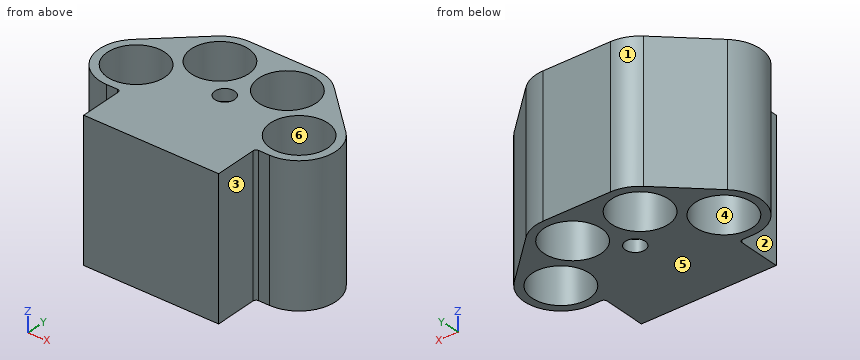
```python
from build123d import *

# Parameters (mm, degrees)
SKETCH1_R           = 7.25
BOSS_EXTRUDE1_DEPTH = 17.5
SKETCH2_R           = 2.5
CUT_EXTRUDE1_DEPTH  = 61.478337768
CUT_EXTRUDE2_START  = -32
SKETCH3_R           = 4
CUT_EXTRUDE2_DEPTH  = 29


with BuildPart() as part:
    # Sketch1 → Boss-Extrude1 (new, symmetric)
    with BuildSketch(Plane.XY):
        with BuildLine():
            ThreePointArc((-20.545709694, 9.528396762), (-29.148813935, 15.380000463), (-26.867170799, 25.531294621))
            Line((-26.867170799, 25.531294621), (-14.821461106, 36.807414431))
            ThreePointArc((-14.821461106, 36.807414431), (-11.898396299, 38.657620814), (-8.5, 39.304516572))
            Line((-8.5, 39.304516572), (0, 39.304516572))
            Line((0, 39.304516572), (0, -2))
            Line((0, -2), (-17, -2))
            Line((-17, -2), (-17, 8.778396762))
            ThreePointArc((-17, 8.778396762), (-17.219669914, 9.308726848), (-17.75, 9.528396762))
            Line((-17.75, 9.528396762), (-20.545709694, 9.528396762))
        make_face()
        with Locations((-8.5, 30.054516572)):
            Circle(SKETCH1_R, mode=Mode.SUBTRACT)
        with Locations((-20.545709694, 18.778396762)):
            Circle(SKETCH1_R, mode=Mode.SUBTRACT)
    boss_extrude1 = extrude(amount=BOSS_EXTRUDE1_DEPTH, both=True)

    # Mirror1: Boss-Extrude1 across plane
    add(boss_extrude1.mirror(Plane(origin=(0, 0, 0), x_dir=(0, 0, 1), z_dir=(1, 0, 0))))

    # Sketch2 → Cut-Extrude1 (cut, through all)
    with BuildSketch(Plane(origin=(0, 0, -17.5), x_dir=(-1, 0, 0), z_dir=(0, 0, -1))):
        with Locations((0, 21)):
            Circle(SKETCH2_R)
    extrude(amount=-CUT_EXTRUDE1_DEPTH, mode=Mode.SUBTRACT)

    # Sketch3 → Cut-Extrude2 (cut)
    with BuildSketch(Plane(origin=(0, 0, -17.5), x_dir=(-1, 0, 0), z_dir=(0, 0, -1)).offset(CUT_EXTRUDE2_START)):
        with Locations((0, 21)):
            Circle(SKETCH3_R)
    extrude(amount=CUT_EXTRUDE2_DEPTH, mode=Mode.SUBTRACT)


solid = part.part
```
Work out the finished part from the listing and answer in its coordinate system (mm). Face numbers are marked on the shaded views. A direction names the side the tool comes from. Round coordinates to 2 decimals unless told otherwise and drop trailing zeros. Loops run counter-clockwise (first coordinate to the right, second up) from the corner with the lowest first, then second, coordinate; pieces in that order, holes last.
(1) The part is cut by section D-D, the plane z = 9. Give the vertices of the cut face in (x, y).
Computed values:
outline: (-26.87, 25.53) arc R9.25 ccw to (-20.55, 9.53) - (-17.75, 9.53) arc R0.75 cw to (-17, 8.78) - (-17, -2) - (17, -2) - (17, 8.78) arc R0.75 cw to (17.75, 9.53) - (20.55, 9.53) arc R9.25 ccw to (26.87, 25.53) - (14.82, 36.81) arc R9.25 ccw to (8.5, 39.3) - (-8.5, 39.3) arc R9.25 ccw to (-14.82, 36.81) - close; hole circle Ø14.5 at (-20.55, 18.78); hole circle Ø14.5 at (-8.5, 30.05); hole circle Ø8 at (0, 21); hole circle Ø14.5 at (8.5, 30.05); hole circle Ø14.5 at (20.55, 18.78)
(2) The mould has two halves that part along X. Classify the marked faces 3, 4, 5 and 6: pulls with the +X half, pulls with the -X half, needs draft (parallel to the pull), parting line crosses it, or undercut.
Computed values:
face 3: pulls with the +X half
face 4: undercut
face 5: needs draft
face 6: undercut
(3) The part is cut by section C-C, the plane y = 21. Give the vertices of the cut face in (x, z).
Computed values:
outline: (-29.52, -17.5) - (-27.45, -17.5) - (-27.45, 17.5) - (-29.52, 17.5) - close; (-13.64, -17.5) - (-2.5, -17.5) - (-2.5, -14.5) - (-4, -14.5) - (-4, 14.5) - (-2.5, 14.5) - (-2.5, 17.5) - (-13.64, 17.5) - close; (2.5, -17.5) - (13.64, -17.5) - (13.64, 17.5) - (2.5, 17.5) - (2.5, 14.5) - (4, 14.5) - (4, -14.5) - (2.5, -14.5) - close; (27.45, -17.5) - (29.52, -17.5) - (29.52, 17.5) - (27.45, 17.5) - close
(4) Each of these flat-tipped pins is pushed along its axis until it touches: P1, Ø4, axis at y = 31.5, z = 10.5, coming from the -X side; P2, Ø12, axis at y = 32.5, z = 9.5, coming from the +X side; P3, Ø1.5, axis at y = 24.5, z = -7.5, coming from the -X side. Where does it stop, or does it pass through?
Computed values:
P1: stops at x = -22.63
P2: stops at x = 25.83
P3: stops at x = -28.35
(5) For the marked faces 1 and 2, determine the directions among +Z, -Z, +X, -X, +Y, -Y from which every point of the face is accessible in a straight line to the end or side of a thin tool.
Computed values:
face 1: +Z, -Z, -X, +Y
face 2: +Z, -Z, -X, -Y
(6) Find the intervals of material crossed by L1, parallel to Y at x = 0, z = 15.15; L2, parallel to X at y = 15.5, z = 7.5; L3, parallel to X at y = 19.5, z = -15, in increasing order.
Computed values:
L1: y = -2 to 18.5, 23.5 to 39.3
L2: x = -29.2 to -27.01, -14.08 to 14.08, 27.01 to 29.2
L3: x = -29.77 to -27.76, -13.33 to -2, 2 to 13.33, 27.76 to 29.77
(7) The part is cut by section B-B, the plane y = 34. Give the vertices of the cut face in (x, z).
Computed values:
outline: (-17.82, -17.5) - (-14.58, -17.5) - (-14.58, 17.5) - (-17.82, 17.5) - close; (-2.42, -17.5) - (2.42, -17.5) - (2.42, 17.5) - (-2.42, 17.5) - close; (14.58, -17.5) - (17.82, -17.5) - (17.82, 17.5) - (14.58, 17.5) - close
(8) The part is cut by section A-A, the plane x = 0. Give the vertices of the cut face in (y, z), and give its area (3 significant figures).
Computed values:
outline: (-2, -17.5) - (18.5, -17.5) - (18.5, -14.5) - (17, -14.5) - (17, 14.5) - (18.5, 14.5) - (18.5, 17.5) - (-2, 17.5) - close; (23.5, -17.5) - (39.3, -17.5) - (39.3, 17.5) - (23.5, 17.5) - (23.5, 14.5) - (25, 14.5) - (25, -14.5) - (23.5, -14.5) - close
area: 1,180 mm2
